Part model, mm, in its own coordinate system. Face numbers are marked on the shaded views. A direction names the side the tool comes from. Round coordinates to 2 decimals unless told otherwise and drop trailing zeros. Loops run counter-clockwise (first coordinate to the right, second up) from the corner with the lowest first, then second, coordinate; pieces in that order, holes last. Notation, with made-up numbers: (-39, 31) - (-33, 31) arc R16 cw to (-33, 38) - close; hole circle Ø9 at (-19.75, -24). An arc over 180 degrees is marked (long way). Put each result on its own line as item: value.
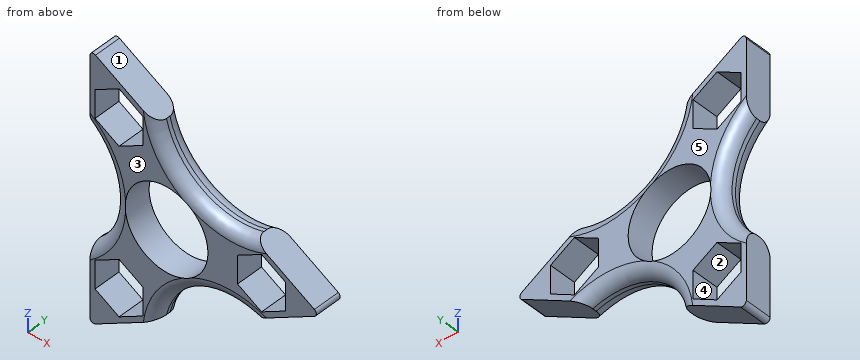
from build123d import *

# Parameters (mm, degrees)
F1_DEPTH = 7
F2_R     = 1
F3_R     = 3
F4_R     = 10.775
F5_DEPTH = 12.5


with BuildPart() as f1:
    # F0 (on Front) → F1 (new body)
    with BuildSketch(Plane.XZ):
        with BuildLine():
            Line((-42.679492, 24.641016), (-60, 34.641016))
            Line((-60, 34.641016), (-60, 14.641016))
            ThreePointArc((-60, 14.641016), (-53.625001, 0), (-60, -14.641016))
            Line((-60, -14.641016), (-60, -34.641016))
            Line((-60, -34.641016), (-42.679492, -24.641016))
            ThreePointArc((-42.679492, -24.641016), (-33.1875, -11.799597), (-17.320508, -10))
            Line((-17.320508, -10), (0, 0))
            Line((0, 0), (-17.320508, 10))
            ThreePointArc((-17.320508, 10), (-33.1875, 11.799597), (-42.679492, 24.641016))
        make_face()
        Polygon((-46.125, -25.042568), (-52.375, -28.651007), (-58.625, -25.042568), (-58.625, -17.82569), (-52.375, -14.21725), (-46.125, -17.82569), align=None, mode=Mode.SUBTRACT)
        Polygon((-46.125, 17.82569), (-52.375, 14.21725), (-58.625, 17.82569), (-58.625, 25.042568), (-52.375, 28.651007), (-46.125, 25.042568), align=None, mode=Mode.SUBTRACT)
        Polygon((-15.25, -7.216878), (-21.5, -3.608439), (-21.5, 3.608439), (-15.25, 7.216878), (-9, 3.608439), (-9, -3.608439), align=None, mode=Mode.SUBTRACT)
    extrude(amount=F1_DEPTH)

    # F2
    f2_edges = [f1.edges().sort_by_distance(p)[0] for p in [
        (-60, -3.5, 34.641016),
        (-60, -3.5, -34.641016),
        (0, -3.5, 0),
    ]]
    fillet(f2_edges, radius=F2_R)

    # F3
    f3_edges = [f1.edges().sort_by_distance(p)[0] for p in [
        (-53.625001, 0, 0),
        (-53.625001, -7, 0),
        (-33.1875, -7, 11.799597),
        (-33.1875, -7, -11.799597),
        (-33.1875, 0, -11.799597),
        (-33.1875, 0, 11.799597),
    ]]
    fillet(f3_edges, radius=F3_R)

    # F4 (on Front) → F5 (cut, symmetric)
    with BuildSketch(Plane.XZ):
        with Locations((-40, 0)):
            Circle(F4_R)
    extrude(amount=F5_DEPTH, both=True, mode=Mode.SUBTRACT)


solid = f1.part
1. Tool access for the marked faces 4 and 5: list every direction of +Z, -Z, +X, -X, +Y, -Y with a clear straight run to the whole face (end or side of a thin tool).
A:
face 4: +Y, -Y
face 5: +Z, -Z, +X, -X, +Y
2. Band-saw the part on C-C (x = -47). List the corners of the cut face in (y, z).
A:
outline: (-7, -27.14) - (0, -27.14) - (0, -25.55) - (-7, -25.55) - close; (-7, -17.32) - (0, -17.32) - (0, -8.19) - (-7, -8.19) - close; (-7, 8.19) - (0, 8.19) - (0, 17.32) - (-7, 17.32) - close; (-7, 25.55) - (0, 25.55) - (0, 27.14) - (-7, 27.14) - close
3. Probe line 1 along X through (y, z) = (-3.25, 0) (3 decimals); line 2 along Z through (x, y) = (-47.5, -5.5); line 3 along X through (y, z) = (-5.5, 0) (3 decimals). List the from-to ranges inside material, lowest first. Write a range as [from, to].
A:
line 1: x = [-53.625, -50.775], [-29.225, -21.5], [-9, -1]
line 2: z = [-27.42, -25.84], [-17.03, -7.74], [7.74, 17.03], [25.84, 27.42]
line 3: x = [-53.223, -50.775], [-29.225, -21.5], [-9, -1]
4. Band-saw the part on A-A (z = 0). List the corners of the cut face in (x, y) (3 decimals), plus the area to 3 significant figures.
A:
outline: (-53.625, -4) arc R3 ccw to (-50.775, -6.996) - (-50.775, -0.004) arc R3 ccw to (-53.625, -3) - close; (-29.225, -7) - (-21.5, -7) - (-21.5, 0) - (-29.225, 0) - close; (-9, -7) - (-1, -7) - (-1, 0) - (-9, 0) - close
area: 126 mm²
5. Two-plate mould, pull along X, no slides. Class the marked faces 1, 2 and 3: pulls with the +X half, pulls with the -X half, needs draft (parallel to the pull), parting line crosses it, or undercut.
A:
face 1: pulls with the +X half
face 2: undercut
face 3: needs draft
6. Pin check, flat tips, straight feed: P1, Ø17, axis at x = -40, z = 0, coming from the +Y side; P2, Ø2, axis at x = -30.5, z = 8.5, coming from the -Y side; P3, Ø3, axis at y = -0.5, z = 4, coming from the +X side; P4, Ø1, axis at x = -49, y = -4, coming from the +Z side. Stop position of each tip, or through.
A:
P1: passes through
P2: stops at y = -7
P3: stops at x = -4.33
P4: stops at z = 28.58
7. Band-saw the part on B-B (y = -4.75). Give the number of separate pieces and of enclosed holes in the cut face, plus the area to 3 significant figures.
A:
separate pieces: 1
enclosed holes: 4
area: 909 mm²
